Input: part model. Units: mm. Frame: model coordinates. A direction names the side the tool comes from. Give positions to 0.01 mm unless a question says otherwise; leave off trailing zeros. Loops run counter-clockwise (first coordinate to the right, second up) from the corner with the lowest first, then second, coordinate; pieces in that order, holes last. Notation, with made-up numbers: (-26, -6.5) - (12, -6.5) arc R32 ccw to (12, 25.5) - close; hole circle Ø10 at (10, -10.75). An arc over 180 degrees is marked (long way). One line per question, with ' | ' between items. Start each with the question number.
from build123d import *

# Parameters (mm, degrees)
SKETCH1_W           = 127
SKETCH1_H           = 50.8
BOSS_EXTRUDE1_DEPTH = 76.2
SKETCH2_R           = 6.75
CUT_EXTRUDE5_DEPTH  = 51.8
SKETCH3_R           = 10.3
CUT_EXTRUDE6_DEPTH  = 13.5


with BuildPart() as part:
    # Sketch1 → Boss-Extrude1 (new body)
    with BuildSketch(Plane(origin=(0, 0, 0), x_dir=(1, 0, 0), z_dir=(0, 1, 0))):
        with Locations((63.5, 25.4)):
            Rectangle(SKETCH1_W, SKETCH1_H)
    extrude(amount=BOSS_EXTRUDE1_DEPTH)

    # Sketch2 → Cut-Extrude5 (cut, through all)
    with BuildSketch(Plane.XY):
        with BuildLine():
            Line((63.5, 38.1), (63.5, 31.35))
            Line((63.5, 31.35), (109.25, 31.35))
            ThreePointArc((109.25, 31.35), (102.5, 38.1), (109.25, 44.85))
            Line((109.25, 44.85), (17.75, 44.85))
            ThreePointArc((17.75, 44.85), (22.522970773, 42.872970773), (24.5, 38.1))
            Line((24.5, 38.1), (63.5, 38.1))
        make_face()
        with BuildLine():
            Line((17.75, 31.35), (63.5, 31.35))
            Line((63.5, 31.35), (63.5, 38.1))
            Line((63.5, 38.1), (24.5, 38.1))
            ThreePointArc((24.5, 38.1), (22.522970773, 33.327029227), (17.75, 31.35))
        make_face()
        with Locations((109.25, 38.1)):
            Circle(SKETCH2_R)
        with BuildLine():
            ThreePointArc((17.75, 44.85), (12.977029227, 42.872970773), (11, 38.1))
            Line((11, 38.1), (24.5, 38.1))
            ThreePointArc((24.5, 38.1), (22.522970773, 42.872970773), (17.75, 44.85))
        make_face()
        with BuildLine():
            Line((24.5, 38.1), (11, 38.1))
            ThreePointArc((11, 38.1), (12.977029227, 33.327029227), (17.75, 31.35))
            ThreePointArc((17.75, 31.35), (22.522970773, 33.327029227), (24.5, 38.1))
        make_face()
    extrude(amount=-CUT_EXTRUDE5_DEPTH, mode=Mode.SUBTRACT)

    # Sketch3 → Cut-Extrude6 (cut)
    with BuildSketch(Plane.XY):
        with BuildLine():
            Line((63.5, 38.1), (63.5, 27.8))
            Line((63.5, 27.8), (110.7, 27.8))
            ThreePointArc((110.7, 27.8), (100.4, 38.099999965), (110.699999929, 48.4))
            Line((110.699999929, 48.4), (16.300000257, 48.4))
            ThreePointArc((16.300000257, 48.4), (23.583199937, 45.383199756), (26.6, 38.1))
            Line((26.6, 38.1), (63.5, 38.1))
        make_face()
        with BuildLine():
            Line((16.3, 27.8), (63.5, 27.8))
            Line((63.5, 27.8), (63.5, 38.1))
            Line((63.5, 38.1), (26.6, 38.1))
            ThreePointArc((26.6, 38.1), (23.583199846, 30.816800154), (16.3, 27.8))
        make_face()
        with BuildLine():
            ThreePointArc((16.300000257, 48.4), (9.016800244, 45.383199937), (6, 38.1))
            Line((6, 38.1), (26.6, 38.1))
            ThreePointArc((26.6, 38.1), (23.583199937, 45.383199756), (16.300000257, 48.4))
        make_face()
        with BuildLine():
            Line((26.6, 38.1), (6, 38.1))
            ThreePointArc((6, 38.1), (9.016800154, 30.816800154), (16.3, 27.8))
            ThreePointArc((16.3, 27.8), (23.583199846, 30.816800154), (26.6, 38.1))
        make_face()
        with Locations((110.7, 38.1)):
            Circle(SKETCH3_R)
    extrude(amount=-CUT_EXTRUDE6_DEPTH, mode=Mode.SUBTRACT)


solid = part.part
Q1. Section A-A, the plane x = 41. Output: boundary loops of the cut face in (y, z).
Q2. Access query for faces 4 (the face through (63, 46, -50.8)), 5 (the face through (62.7, 45.1, -13.5)), 6 (the face through (64, 44.85, -32)). Directions: +Z, -Z, +X, -X, +Y, -Y. A direction counts if a zero-diameter tool reaches every point of the face in a straight line with its end or side. Return the directions, or none.
Q3. Line query: L1, parallel to Y at x = 102, z = -10.5; L2, parallel to Y at x = 91.5, z = -49; L3, parallel to X at y = 43, z = -7. Output: solid intervals per line, ascending. Write a range as from..to.
Q4. Section C-C, the plane z = -4.5. Output: boundary loops of the cut face in (x, y).
Q5. Draft query along X for faces 1 (the face through (63, 76.2, -26)), 2 (the face through (63, 31.35, -32)), 3 (the face through (0, 38, -25)). Return one class per face: +X half, -X half, draft (parallel to the pull), parting line (faces both ways), or undercut.
Q6. Section B-B, the plane z = -40.5. Output: boundary loops of the cut face in (x, y), plus the area to 3 significant figures.
Solved:
1) outline: (0, -50.8) - (31.35, -50.8) - (31.35, -13.5) - (27.8, -13.5) - (27.8, 0) - (0, 0) - close; (44.85, -50.8) - (76.2, -50.8) - (76.2, 0) - (48.4, 0) - (48.4, -13.5) - (44.85, -13.5) - close
2) face 4: -Z, +X, -X, +Y, -Y | face 5: +Z | face 6: +Z, -Z
3) L1: y = 0..27.8, 48.4..76.2 | L2: y = 0..31.35, 44.85..76.2 | L3: x = 0..7.24, 119.76..127
4) outline: (0, 0) - (127, 0) - (127, 76.2) - (0, 76.2) - close; hole (16.3, 27.8) - (110.7, 27.8) arc R10.3 ccw to (110.7, 48.4) - (16.3, 48.4) arc R10.3 ccw to start
5) face 1: draft | face 2: undercut | face 3: -X half
6) outline: (0, 0) - (127, 0) - (127, 76.2) - (0, 76.2) - close; hole (17.75, 31.35) - (109.25, 31.35) arc R6.75 ccw to (109.25, 44.85) - (17.75, 44.85) arc R6.75 ccw to start | area: 8,300 mm²
